Model file for the job. Use its own axes, mm. Face numbers are marked on the shaded views. A direction names the side the tool comes from. Give positions to 0.01 mm unless a question says otherwise; leave off trailing zeros. Order: outer loops, then holes, each group sorted by start corner. A loop starts at its lowest first (then second) coordinate and runs counter-clockwise, first axis right, second up. Notation, with made-up numbers: M -23.5,70 L 9.5,70 A22 ccw 9.5,93 Z; hole C 58,36.5 d1. An arc over 180 degrees is marked long. Return JSON: item names as keys, results as strings. Group by question number.
1. Slice it at B-B on x = -21. List the corners of the cut face in (y, z), then the cut area to 3 significant figures.
2. 3-axis set-ups, long thin cutter, end or side, ignore diameter. For the marked faces 4, 5 and 6: which of +Z, -Z, +X, -X, +Y, -Y reach the whole face in a straight line?
3. Slice it at A-A on z = -24.5. List the corners of the cut face in (x, y), then the cut area to 3 significant figures.
4. Wall check: probe 1 along X at (y, z) = (4.5, -23.5); probe 2 along Z at (x, y) = (-27.25, 2.5); probe 3 along Z at (x, y) = (-20.25, 3). Give the ranges that are in metal, low to high. Write a range as [from, to].
5. Slice it at D-D on z = -27.5. List the corners of the cut face in (x, y), then the cut area to 3 significant figures.
6. Pin check, flat tips, straight feed: pin 1 (0.9 mm diameter, centred on y = -2, z = -23, fed in from +X); pin 2 (0.9 mm diameter, centred on y = 5, z = -23, fed in from -X). Stop position of each tip, or through.
7. Slice it at C-C on y = -0.75. Give the number of separate pieces and of enclosed holes in the cut face, then the cut area to 3 significant figures.
8. Two-plate mould, pull along Z, no slides. Class the marked faces 1, 2 and 3: released by +Z, released by -Z, zero draft, split by the parting line, or undercut.
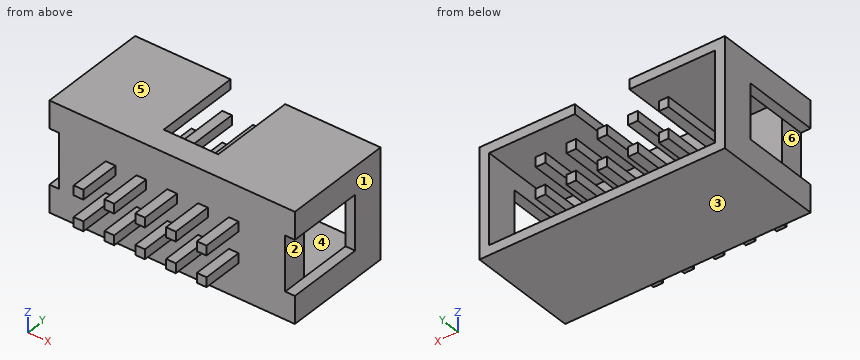
from build123d import *

# Parameters (mm, degrees)
SKETCH1_W           = 20.25
SKETCH1_H           = 9
BOSS_EXTRUDE1_DEPTH = 9.1
SKETCH2_W           = 18.65
SKETCH2_H           = 7.4
CUT_EXTRUDE1_DEPTH  = 7.1
SKETCH2_3_W         = 0.8
SKETCH2_3_H         = 0.8
BOSS_EXTRUDE2_DEPTH = 12.5
SKETCH3_W           = 4.5
SKETCH3_H           = 7.1
CUT_EXTRUDE2_DEPTH  = 2.1
SKETCH5_W           = 4.5
SKETCH5_H           = 6.4
CUT_EXTRUDE3_DEPTH  = 0.8
SKETCH6_W           = 4.5
SKETCH6_H           = 6.4
CUT_EXTRUDE4_DEPTH  = 0.8


with BuildPart() as part:
    # Sketch1 → Boss-Extrude1 (new body)
    with BuildSketch(Plane(origin=(0, 0, 0), x_dir=(1, 0, 0), z_dir=(0, 1, 0))):
        with Locations((-29.615572658, 24.590099186)):
            Rectangle(SKETCH1_W, SKETCH1_H)
    extrude(amount=BOSS_EXTRUDE1_DEPTH)

    # Sketch2 → Cut-Extrude1 (cut)
    with BuildSketch(Plane(origin=(0, 9.1, 0), x_dir=(1, 0, 0), z_dir=(0, 1, 0))):
        with Locations((-29.615572658, 24.590099186)):
            Rectangle(SKETCH2_W, SKETCH2_H)
    extrude(amount=-CUT_EXTRUDE1_DEPTH, mode=Mode.SUBTRACT)

    # Sketch2<3> → Boss-Extrude2 (add)
    with BuildSketch(Plane(origin=(0, 9.1, 0), x_dir=(1, 0, 0), z_dir=(0, 1, 0))):
        with Locations((-32.155572658, 23.320099186)):
            Rectangle(SKETCH2_3_W, SKETCH2_3_H)
        with Locations((-29.615572658, 23.320099186)):
            Rectangle(SKETCH2_3_W, SKETCH2_3_H)
        with Locations((-27.075572658, 23.320099186)):
            Rectangle(SKETCH2_3_W, SKETCH2_3_H)
        with Locations((-24.535572658, 23.320099186)):
            Rectangle(SKETCH2_3_W, SKETCH2_3_H)
        with Locations((-29.615572658, 25.860099186)):
            Rectangle(SKETCH2_3_W, SKETCH2_3_H)
        with Locations((-27.075572658, 25.860099186)):
            Rectangle(SKETCH2_3_W, SKETCH2_3_H)
        with Locations((-24.535572658, 25.860099186)):
            Rectangle(SKETCH2_3_W, SKETCH2_3_H)
        with Locations((-32.155572658, 25.860099186)):
            Rectangle(SKETCH2_3_W, SKETCH2_3_H)
        with Locations((-34.695572658, 23.320099186)):
            Rectangle(SKETCH2_3_W, SKETCH2_3_H)
        with Locations((-34.695572658, 25.860099186)):
            Rectangle(SKETCH2_3_W, SKETCH2_3_H)
    extrude(amount=-BOSS_EXTRUDE2_DEPTH)

    # Sketch3 → Cut-Extrude2 (cut)
    with BuildSketch(Plane.XY.offset(-20.090099186)):
        with Locations((-29.615572658, 5.55)):
            Rectangle(SKETCH3_W, SKETCH3_H)
    extrude(amount=-CUT_EXTRUDE2_DEPTH, mode=Mode.SUBTRACT)

    # Sketch5 → Cut-Extrude3 (cut)
    with BuildSketch(Plane.ZY.offset(39.740572658)):
        with Locations((-24.590099186, 3.2)):
            Rectangle(SKETCH5_W, SKETCH5_H)
    extrude(amount=-CUT_EXTRUDE3_DEPTH, mode=Mode.SUBTRACT)

    # Sketch6 → Cut-Extrude4 (cut)
    with BuildSketch(Plane(origin=(-19.490572658, 0, 0), x_dir=(0, 0, -1), z_dir=(1, 0, 0))):
        with Locations((24.590099186, 3.2)):
            Rectangle(SKETCH6_W, SKETCH6_H)
    extrude(amount=-CUT_EXTRUDE4_DEPTH, mode=Mode.SUBTRACT)


solid = part.part
Result:
{
 "1": {"outline": "M 0,-29.09 L 9.1,-29.09 L 9.1,-28.29 L 2,-28.29 L 2,-20.89 L 9.1,-20.89 L 9.1,-20.09 L 0,-20.09 Z", "area": "29.4 mm2"},
 "2": {"face 4": "+Y", "face 5": "+Z, +X, -X, +Y, -Y", "face 6": "-X, -Y"},
 "3": {"outline": "M -39.74,6.4 L -38.94,6.4 L -38.94,9.1 L -39.74,9.1 Z; M -38.94,0 L -20.29,0 L -20.29,2 L -38.94,2 Z; M -20.29,6.4 L -19.49,6.4 L -19.49,9.1 L -20.29,9.1 Z", "area": "41.6 mm2"},
 "4": {"probe 1": "x = [-35.1, -34.3], [-32.56, -31.76], [-30.02, -29.22], [-27.48, -26.68], [-24.94, -24.14]", "probe 2": "z = [-29.09, -28.29], [-26.26, -25.46], [-23.72, -22.92], [-20.89, -20.09]", "probe 3": "z = [-29.09, -26.84], [-22.34, -20.09]"},
 "5": {"outline": "M -39.74,0 L -19.49,0 L -19.49,9.1 L -20.29,9.1 L -20.29,2 L -38.94,2 L -38.94,9.1 L -39.74,9.1 Z", "area": "51.9 mm2"},
 "6": {"pin 1": "stops at x = -24.14", "pin 2": "stops at x = -35.1"},
 "7": {"separate pieces": "10", "enclosed holes": "0", "area": "6.40 mm2"},
 "8": {"face 1": "zero draft", "face 2": "undercut", "face 3": "released by -Z"}
}
